Geometry check sheet. Reference: the model listing, model coordinates, mm. A direction names the side the tool comes from. Coordinates: 2 decimals unless noted, no trailing zeros. Order: outer loops, then holes, each group sorted by start corner. A loop starts at its lowest first (then second) coordinate and runs counter-clockwise, first axis right, second up. Notation, with made-up numbers: (52, 78.25) - (81, 78.25) arc R35 ccw to (81, 112.25) - close; hole circle Ø5 at (89, -12.75). An arc over 180 degrees is marked (long way). Put each result on its own line as item: value.
from build123d import *

# Parameters (mm, degrees)
BOSS_EXTRUDE1_START  = 66.4
SKETCH1_R            = 9
BOSS_EXTRUDE1_DEPTH  = 4
BOSS_EXTRUDE2_START  = 60
SKETCH2_W            = 4
SKETCH2_H            = 55
BOSS_EXTRUDE2_DEPTH  = 12
BOSS_EXTRUDE3_START  = 41.1
SKETCH3_W            = 4
SKETCH3_H            = 18.5
BOSS_EXTRUDE3_DEPTH  = 39
BOSS_EXTRUDE4_START  = 65.4
BOSS_EXTRUDE4_DEPTH  = 6
BOSS_EXTRUDE5_START  = 65.4
BOSS_EXTRUDE5_DEPTH  = 6
BOSS_EXTRUDE6_START  = 65.9
SKETCH6_R            = 4.6
BOSS_EXTRUDE6_DEPTH  = 2.3
BOSS_EXTRUDE7_START  = 62.7
SKETCH7_W            = 2.3
SKETCH7_H            = 17.5
BOSS_EXTRUDE7_DEPTH  = 6.6
BOSS_EXTRUDE8_START  = 65.1
SKETCH8_W            = 6
SKETCH8_H            = 10.5
BOSS_EXTRUDE8_DEPTH  = 1.8
BOSS_EXTRUDE9_START  = 62.7
SKETCH9_W            = 2.3
SKETCH9_H            = 17.5
BOSS_EXTRUDE9_DEPTH  = 6.6
BOSS_EXTRUDE10_START = 65.1
SKETCH10_W           = 6
SKETCH10_H           = 10.5
BOSS_EXTRUDE10_DEPTH = 1.8
BOSS_EXTRUDE11_START = 65.4
SKETCH11_R           = 3
BOSS_EXTRUDE11_DEPTH = 6
BOSS_EXTRUDE12_START = 48.9
SKETCH12_W           = 6
SKETCH12_H           = 13
BOSS_EXTRUDE12_DEPTH = 23.4
BOSS_EXTRUDE13_START = 45.075
SKETCH13_W           = 6
SKETCH13_H           = 2
BOSS_EXTRUDE13_DEPTH = 2.9
BOSS_EXTRUDE14_START = 73.225
SKETCH14_W           = 6
SKETCH14_H           = 2
BOSS_EXTRUDE14_DEPTH = 2.9


with BuildPart() as part:
    # Sketch1 → Boss-Extrude1 (new body)
    with BuildSketch(Plane(origin=(0, 0, 0), x_dir=(0, 0, -1), z_dir=(1, 0, 0)).offset(BOSS_EXTRUDE1_START)):
        with Locations((-66, -20)):
            Circle(SKETCH1_R)
    extrude(amount=BOSS_EXTRUDE1_DEPTH)

    # Sketch2 → Boss-Extrude2 (add)
    with BuildSketch(Plane.XY.offset(BOSS_EXTRUDE2_START)):
        with Locations((68.4, -28.5)):
            Rectangle(SKETCH2_W, SKETCH2_H)
    extrude(amount=BOSS_EXTRUDE2_DEPTH)

    # Sketch3 → Boss-Extrude3 (add)
    with BuildSketch(Plane.XY.offset(BOSS_EXTRUDE3_START)):
        with Locations((68.4, -64.25)):
            Rectangle(SKETCH3_W, SKETCH3_H)
    extrude(amount=BOSS_EXTRUDE3_DEPTH)


with BuildPart() as body_2:
    # Sketch4 → Boss-Extrude4 (new body)
    with BuildSketch(Plane(origin=(0, 0, 0), x_dir=(0, 0, -1), z_dir=(1, 0, 0)).offset(BOSS_EXTRUDE4_START)):
        Polygon((-81.1, -74.5), (-73.1, -74.5), (-81.1, -66.5), align=None)
    extrude(amount=BOSS_EXTRUDE4_DEPTH)


with BuildPart() as part_1:
    add(part.part)

    # Combine1: cut body 2
    add(body_2.part, mode=Mode.SUBTRACT)


with BuildPart() as body_2_2:
    # Sketch5 → Boss-Extrude5 (new body)
    with BuildSketch(Plane(origin=(0, 0, 0), x_dir=(0, 0, -1), z_dir=(1, 0, 0)).offset(BOSS_EXTRUDE5_START)):
        Polygon((-40.1, -74.5), (-48.1, -74.5), (-40.1, -66.5), align=None)
    extrude(amount=BOSS_EXTRUDE5_DEPTH)


with BuildPart() as part_2:
    add(part_1.part)

    # Combine2: cut body 2 2
    add(body_2_2.part, mode=Mode.SUBTRACT)


with BuildPart() as body_2_3:
    # Sketch6 → Boss-Extrude6 (new body)
    with BuildSketch(Plane(origin=(0, 0, 0), x_dir=(0, 0, -1), z_dir=(1, 0, 0)).offset(BOSS_EXTRUDE6_START)):
        with Locations((-66, -20)):
            Circle(SKETCH6_R)
    extrude(amount=BOSS_EXTRUDE6_DEPTH)


with BuildPart() as part_3:
    add(part_2.part)

    # Combine3: cut body 2 3
    add(body_2_3.part, mode=Mode.SUBTRACT)


with BuildPart() as body_2_4:
    # Sketch7 → Boss-Extrude7 (new body)
    with BuildSketch(Plane.XY.offset(BOSS_EXTRUDE7_START)):
        with Locations((67.05, -11.25)):
            Rectangle(SKETCH7_W, SKETCH7_H)
    extrude(amount=BOSS_EXTRUDE7_DEPTH)


with BuildPart() as part_4:
    add(part_3.part)

    # Combine4: cut body 2 4
    add(body_2_4.part, mode=Mode.SUBTRACT)


with BuildPart() as body_2_5:
    # Sketch8 → Boss-Extrude8 (new body)
    with BuildSketch(Plane.XY.offset(BOSS_EXTRUDE8_START)):
        with Locations((68.4, -9.25)):
            Rectangle(SKETCH8_W, SKETCH8_H)
    extrude(amount=BOSS_EXTRUDE8_DEPTH)


with BuildPart() as part_5:
    add(part_4.part)

    # Combine5: cut body 2 5
    add(body_2_5.part, mode=Mode.SUBTRACT)


with BuildPart() as body_2_6:
    # Sketch9 → Boss-Extrude9 (new body)
    with BuildSketch(Plane.XY.offset(BOSS_EXTRUDE9_START)):
        with Locations((67.05, -28.75)):
            Rectangle(SKETCH9_W, SKETCH9_H)
    extrude(amount=BOSS_EXTRUDE9_DEPTH)


with BuildPart() as part_6:
    add(part_5.part)

    # Combine6: cut body 2 6
    add(body_2_6.part, mode=Mode.SUBTRACT)


with BuildPart() as body_2_7:
    # Sketch10 → Boss-Extrude10 (new body)
    with BuildSketch(Plane.XY.offset(BOSS_EXTRUDE10_START)):
        with Locations((68.4, -30.75)):
            Rectangle(SKETCH10_W, SKETCH10_H)
    extrude(amount=BOSS_EXTRUDE10_DEPTH)


with BuildPart() as part_7:
    add(part_6.part)

    # Combine7: cut body 2 7
    add(body_2_7.part, mode=Mode.SUBTRACT)


with BuildPart() as body_2_8:
    # Sketch11 → Boss-Extrude11 (new body)
    with BuildSketch(Plane(origin=(0, 0, 0), x_dir=(0, 0, -1), z_dir=(1, 0, 0)).offset(BOSS_EXTRUDE11_START)):
        with Locations((-66, -20)):
            Circle(SKETCH11_R)
    extrude(amount=BOSS_EXTRUDE11_DEPTH)


with BuildPart() as part_8:
    add(part_7.part)

    # Combine8: cut body 2 8
    add(body_2_8.part, mode=Mode.SUBTRACT)


with BuildPart() as body_2_9:
    # Sketch12 → Boss-Extrude12 (new body)
    with BuildSketch(Plane.XY.offset(BOSS_EXTRUDE12_START)):
        with Locations((68.4, -65)):
            Rectangle(SKETCH12_W, SKETCH12_H)
    extrude(amount=BOSS_EXTRUDE12_DEPTH)


with BuildPart() as part_9:
    add(part_8.part)

    # Combine9: cut body 2 9
    add(body_2_9.part, mode=Mode.SUBTRACT)


with BuildPart() as body_2_10:
    # Sketch13 → Boss-Extrude13 (new body)
    with BuildSketch(Plane.XY.offset(BOSS_EXTRUDE13_START)):
        with Locations((68.4, -65)):
            Rectangle(SKETCH13_W, SKETCH13_H)
    extrude(amount=BOSS_EXTRUDE13_DEPTH)


with BuildPart() as part_10:
    add(part_9.part)

    # Combine10: cut body 2 10
    add(body_2_10.part, mode=Mode.SUBTRACT)


with BuildPart() as body_2_11:
    # Sketch14 → Boss-Extrude14 (new body)
    with BuildSketch(Plane.XY.offset(BOSS_EXTRUDE14_START)):
        with Locations((68.4, -65)):
            Rectangle(SKETCH14_W, SKETCH14_H)
    extrude(amount=BOSS_EXTRUDE14_DEPTH)


with BuildPart() as part_11:
    add(part_10.part)

    # Combine11: cut body 2 11
    add(body_2_11.part, mode=Mode.SUBTRACT)


solid = part_11.part
Q1. Section check A-A on y = -9.5. Record the boundary of the cut face in (x, z).
Answer block:
outline: (66.4, 60) - (70.4, 60) - (70.4, 65.1) - (68.2, 65.1) - (68.2, 62.7) - (66.4, 62.7) - close; (66.4, 69.3) - (68.2, 69.3) - (68.2, 66.9) - (70.4, 66.9) - (70.4, 72) - (66.4, 72) - close
Q2. Depth check by flat-ended pin: pin 1 Ø0.9 at (x, y) = (67, -12) entering from +Z; pin 2 Ø0.9 at (x, z) = (68, 46.5) entering from -Y; pin 3 Ø1.4 at (x, y) = (67, -11.5) entering from -Z. Enter the tip coordinate at first touch or a pass-through.
Answer block:
pin 1: stops at z = 72
pin 2: stops at y = -73.35
pin 3: stops at z = 60
Q3. Section check C-C on x = 67.3. State how many separate pieces and enclosed holes the cut face has, then the cut area to 3 significant figures.
Answer block:
separate pieces: 1
enclosed holes: 4
area: 831 mm^2
Q4. Thickness scan on L1, parallel to Y at x = 69.65, z = 66; L2, parallel to Y at x = 66.95, z = 66; L3, parallel to Y at x = 68, z = 52. Record the ranges inside material, lowest first. Write a range as [from, to].
Answer block:
L1: y = [-73.5, -71.5], [-58.5, -36], [-25.5, -23], [-17, -14.5], [-4, -1]
L2: y = [-73.5, -71.5], [-58.5, -37.5], [-2.5, -1]
L3: y = [-73.5, -71.5], [-58.5, -55]
Q5. Section check B-B on z = 66. Record the boundary of the cut face in (x, y), then the cut area to 3 significant figures.
Answer block:
outline: (66.4, -73.5) - (70.4, -73.5) - (70.4, -71.5) - (66.4, -71.5) - close; (66.4, -58.5) - (70.4, -58.5) - (70.4, -36) - (68.2, -36) - (68.2, -37.5) - (66.4, -37.5) - close; (66.4, -2.5) - (68.2, -2.5) - (68.2, -4) - (70.4, -4) - (70.4, -1) - (66.4, -1) - close; (68.2, -25.5) - (70.4, -25.5) - (70.4, -23) - (68.2, -23) - close; (68.2, -17) - (70.4, -17) - (70.4, -14.5) - (68.2, -14.5) - close
area: 116 mm^2
Q6. Section check D-D on z = 55.5. Record the boundary of the cut face in (x, y).
Answer block:
outline: (66.4, -73.5) - (70.4, -73.5) - (70.4, -71.5) - (66.4, -71.5) - close; (66.4, -58.5) - (70.4, -58.5) - (70.4, -55) - (66.4, -55) - close
Q7. Access from +Z, -Z, +X, -X, +Y, -Y to the whole of each face (thin tool, end or side, straight path). Record for faces 4 (the flat face through (68, -7, 60)), 5 (the flat face through (68, -41, 60)), 6 (the flat face through (67, -2.5, 66)), 7 (the flat face through (68, -65, 48.9)), 8 (the flat face through (68, -55, 76)).
Answer block:
face 4: -Z, +X, -X, +Y
face 5: -Z, +X, -X
face 6: -X
face 7: +X, -X
face 8: +Z, +X, -X
Q8. Draft check along Z on faces 1 (the flat face through (68.4, -70.5, 44.1)), 2 (the flat face through (67, -30, 62.7)), 3 (the flat face through (70.4, -40, 63)). Enter one of: pulls with the +Z half, pulls with the -Z half, needs draft (parallel to the pull), parting line crosses it, or undercut.
Answer block:
face 1: pulls with the -Z half
face 2: undercut
face 3: needs draft
